Here's how the part is built. I have some questions about the finished solid (model axes, mm). Round coordinates to 2 decimals unless told otherwise and drop trailing zeros. Write each loop counter-clockwise with the first axis right and the second up, starting at its lowest first coordinate (ties: lowest second). Pieces come first, ordered by that corner, then holes. Notation, with made-up numbers: M -16.75,38.5 L 8.25,38.5 A24 ccw 8.25,52.5 Z; hole C 44.25,15.25 d1. An arc over 180 degrees is marked long. Write item = value, one per line. Start each with the question number.
(1) I need wall thicknesses on line 1 along Y through (x, z) = (0, 3.9); line 2 along Y through (x, z) = (75, 1.6); line 3 along X through (y, z) = (-50, 3.9). Which ranges of each line are inside material? Lowest first, please.
(2) I want a section at B-B (y = -51.4). List the corners of the cut face in (x, z) for me, and give its area (3 significant figures).
(3) Will these pins go through, and if not, where does the flat tip stop? pin 1 Ø2 at (x, y) = (31.5, -6.5) entering from -Z; pin 2 Ø2 at (x, z) = (-12.5, 4) entering from +Y; pin 3 Ø4.5 at (x, y) = (-75, -51.4) entering from +Z.
(4) I want a section at A-A (x = -75). List the corners of the cut face in (y, z) for me.
(5) I want a section at C-C (z = 3.2). List the corners of the cut face in (x, y) for me, and give its area (3 significant figures).
(6) I want a section at D-D (y = 43.5). List the corners of the cut face in (x, z) for me, and give its area (3 significant figures).
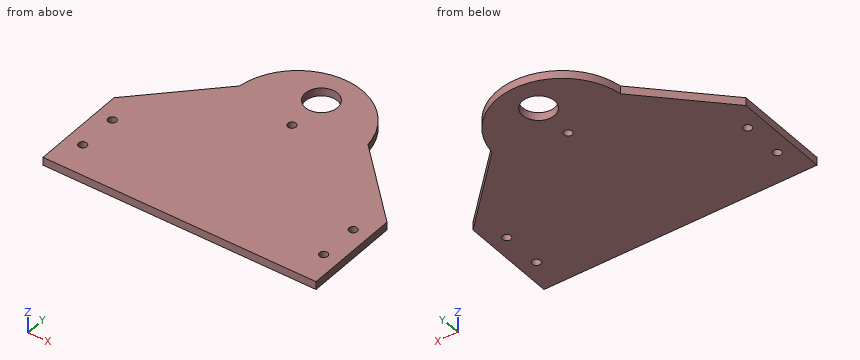
```python
from build123d import *

# Parameters (mm, degrees)
SKETCH_1_R      = 2.55
SKETCH_1_R_2    = 10
EXTRUDE_1_DEPTH = 5


with BuildPart() as part:
    # ｽｹｯﾁ1 → ﾎﾞｽ - 押し出し1 (new body)
    with BuildSketch(Plane.XY):
        with BuildLine():
            Line((-85, -71.4), (-85, -11.4))
            Line((-85, -11.4), (-40, 33.6))
            ThreePointArc((-40, 33.6), (0, 68.911288741), (40, 33.6))
            Line((40, 33.6), (85, -11.4))
            Line((85, -11.4), (85, -71.4))
            Line((85, -71.4), (-85, -71.4))
        make_face()
        with Locations((75, -26.4)):
            Circle(SKETCH_1_R, mode=Mode.SUBTRACT)
        with Locations((75, -51.4)):
            Circle(SKETCH_1_R, mode=Mode.SUBTRACT)
        with Locations((-75, -26.4)):
            Circle(SKETCH_1_R, mode=Mode.SUBTRACT)
        with Locations((-75, -51.4)):
            Circle(SKETCH_1_R, mode=Mode.SUBTRACT)
        with Locations((0, 23.6)):
            Circle(SKETCH_1_R, mode=Mode.SUBTRACT)
        with Locations((0, 48.6)):
            Circle(SKETCH_1_R_2, mode=Mode.SUBTRACT)
    extrude(amount=EXTRUDE_1_DEPTH)


solid = part.part
```
Returned:
q1.line_1 = -71.4 to 21.05, 26.15 to 38.6, 58.6 to 68.91
q1.line_2 = -71.4 to -53.95, -48.85 to -28.95, -23.85 to -1.4
q1.line_3 = -85 to -77.13, -72.87 to 72.87, 77.13 to 85
q2.outline = M -85,0 L -77.55,0 L -77.55,5 L -85,5 Z; M -72.45,0 L 72.45,0 L 72.45,5 L -72.45,5 Z; M 77.55,0 L 85,0 L 85,5 L 77.55,5 Z
q2.area = 799 mm²
q3.pin_1 = 0
q3.pin_2 = 67.24
q3.pin_3 = through
q4.outline = M -71.4,0 L -53.95,0 L -53.95,5 L -71.4,5 Z; M -48.85,0 L -28.95,0 L -28.95,5 L -48.85,5 Z; M -23.85,0 L -1.4,0 L -1.4,5 L -23.85,5 Z
q5.outline = M -85,-71.4 L 85,-71.4 L 85,-11.4 L 40,33.6 A40.31 ccw -40,33.6 L -85,-11.4 Z; hole C -75,-51.4 d5.1; hole C -75,-26.4 d5.1; hole C 0,48.6 d20; hole C 0,23.6 d5.1; hole C 75,-51.4 d5.1; hole C 75,-26.4 d5.1
q5.area = 17,600 mm²
q6.outline = M -37.46,0 L -8.6,0 L -8.6,5 L -37.46,5 Z; M 8.6,0 L 37.46,0 L 37.46,5 L 8.6,5 Z
q6.area = 289 mm²
